Design review of the part built by this model. Coordinates are the model's own, in mm. Give positions to 0.01 mm unless a question says otherwise; leave off trailing zeros. Write each loop counter-clockwise with the first axis right and the second up, starting at its lowest first coordinate (ties: lowest second). Pieces come first, ordered by that corner, then holes. Notation, with made-up numbers: (27.5, 68) -> (35.5, 68) arc R30 cw to (35.5, 107) -> close; hole circle Ø8 at (82, 71). An arc over 180 degrees is marked (long way). Return JSON: item names as keys, results as strings. Group by question number.
Autodesk Inventor part; units mm, degrees
ref_plane "YZ Plane" through (0, 0, 0) normal (1, 0, 0) x (0, 1, 0)
ref_plane "XZ Plane" through (0, 0, 0) normal (0, 1, 0) x (-1, 0, 0)
ref_plane "XY Plane" through (0, 0, 0) normal (0, 0, 1) x (1, 0, 0)
sketch "Sketch1" plane through (0, 0, 0) normal (1, 0, 0) x (0, 1, 0)
  circle A0 centre (0, 0) radius 71
  dimension "d0" = 142
extrude "Extrusion1" add sketch "Sketch1" along normal blind 150
sketch "Sketch2" plane through (150, 0, 0) normal (1, 0, 0) x (0, 0, -1)
  line L0 (0, 0) -> (0, -44.2)
  circle A0 centre (0, 0) radius 71
  line L1 (-55.564, -44.2) -> (55.564, -44.2)
  dimension "d3" = 44.2
extrude "Extrusion2" cut sketch "Sketch2" against normal blind 150 contours A0 L1 picked at (-0.2063, 32.437)
sketch "Sketch3" plane through (150, 0, 0) normal (1, 0, 0) x (0, 0, -1)
  line L0 (0, 0) -> (0, -64.2)
  arc A0 (-55.564, -44.2) -> (55.564, -44.2) centre (0, 0) ccw
  line L1 (-30.3209, -64.2) -> (30.3209, -64.2)
  dimension "d6" = 64.2
sketch "Sketch5" plane through (150, -44.2, 55.564) normal (0, 1, 0) x (1, 0, 0)
  line L0 (-150, 55.564) -> (-75, 55.564)
  line L1 (-75, 55.564) -> (-75, 68.264)
  line L2 (-75, 55.564) -> (-75, 42.864)
  circle A0 centre (-75, 68.264) radius 3
  circle A1 centre (-75, 42.864) radius 3
  line L3 (-75, 68.264) -> (-49.6, 68.264)
  line L4 (-75, 42.864) -> (-49.6, 42.864)
  line L5 (-75, 68.264) -> (-100.4, 68.264)
  line L6 (-75, 42.864) -> (-100.4, 42.864)
  circle A2 centre (-100.4, 68.264) radius 3
  circle A3 centre (-49.6, 68.264) radius 3
  circle A4 centre (-49.6, 42.864) radius 3
  circle A5 centre (-100.4, 42.864) radius 3
  line L7 (-100.4, 42.864) -> (-125.8, 42.864)
  line L8 (-100.4, 68.264) -> (-125.8, 68.264)
  line L9 (-49.6, 68.264) -> (-24.2, 68.264)
  line L10 (-49.6, 42.864) -> (-24.2, 42.864)
  circle A6 centre (-125.8, 68.264) radius 3
  circle A7 centre (-125.8, 42.864) radius 3
  circle A8 centre (-24.2, 68.264) radius 3
  circle A9 centre (-24.2, 42.864) radius 3
  line L11 (-125.8, 68.264) -> (-125.8, 93.664)
  line L12 (-100.4, 68.264) -> (-100.4, 93.664)
  line L13 (-75, 68.264) -> (-75, 93.664)
  line L14 (-75, 68.264) -> (-49.6, 68.264) construction
  line L15 (-49.6, 68.264) -> (-49.6, 93.664)
  line L16 (-24.2, 68.264) -> (-24.2, 93.664)
  line L17 (-125.8, 42.864) -> (-125.8, 17.464)
  line L18 (-100.4, 42.864) -> (-100.4, 17.464)
  line L19 (-75, 42.864) -> (-75, 17.464)
  line L20 (-49.6, 42.864) -> (-49.6, 17.464)
  line L21 (-24.2, 42.864) -> (-24.2, 17.464)
  circle A10 centre (-125.8, 93.664) radius 3
  circle A11 centre (-100.4, 93.664) radius 3
  circle A12 centre (-75, 93.664) radius 3
  circle A13 centre (-49.6, 93.664) radius 3
  circle A14 centre (-24.2, 93.664) radius 3
  circle A15 centre (-24.2, 17.464) radius 3
  circle A16 centre (-49.6, 17.464) radius 3
  circle A17 centre (-75, 17.464) radius 3
  circle A18 centre (-100.4, 17.464) radius 3
  circle A19 centre (-125.8, 17.464) radius 3
  dimension "d9" = 75
  dimension "d10" = 12.7
  dimension "d11" = 12.7
  dimension "d12" = 6
  dimension "d13" = 6
  dimension "d14" = 25.4
  dimension "d15" = 25.4
  dimension "d16" = 25.4
  dimension "d17" = 25.4
  dimension "d18" = 6
  dimension "d19" = 6
  dimension "d20" = 6
  dimension "d21" = 6
  dimension "d22" = 25.4
  dimension "d23" = 25.4
  dimension "d24" = 25.4
  dimension "d25" = 25.4
  dimension "d26" = 6
  dimension "d27" = 6
  dimension "d28" = 6
  dimension "d29" = 6
  dimension "d30" = 25.4
  dimension "d31" = 25.4
  dimension "d32" = 25.4
  dimension "d33" = 90
  dimension "d34" = 25.4
  dimension "d35" = 25.4
  dimension "d36" = 25.4
  dimension "d37" = 25.4
  dimension "d38" = 25.4
  dimension "d39" = 25.4
  dimension "d40" = 25.4
  dimension "d41" = 6
  dimension "d42" = 6
  dimension "d43" = 6
  dimension "d44" = 6
  dimension "d45" = 6
  dimension "d46" = 6
  dimension "d47" = 6
  dimension "d48" = 6
  dimension "d49" = 6
  dimension "d50" = 6
sketch "Sketch6" plane through (150, 0, 0) normal (1, 0, 0) x (0, 0, -1)
  point P0 (0, 0)
extrude "Extrusion4" cut sketch "Sketch3" against normal blind 150
extrude "Extrusion5" cut sketch "Sketch5" against normal blind 10
thread "Thread1"
thread "Thread2"
thread "Thread3"
thread "Thread4"
thread "Thread5"
thread "Thread6"
thread "Thread7"
thread "Thread8"
thread "Thread9"
thread "Thread10"
thread "Thread11"
thread "Thread12"
thread "Thread13"
thread "Thread14"
thread "Thread15"
thread "Thread16"
thread "Thread17"
thread "Thread18"
thread "Thread19"
thread "Thread20"
properties part number "Base"
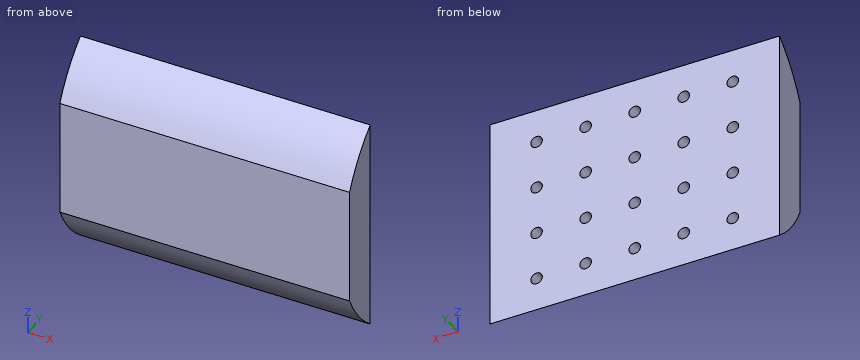
Q1. Take a section at C-C, the plane z = 12.7. Give the boundary of the cut face in (x, y).
Q2. For L1, parallel to X at y = -46.75, z = -38.1; L2, parallel to Z at x = 125.8, y = -48.5; L3, parallel to Z at x = 100.4, y = -46.5, list the stretches that pass through material, from the lowest coordinate up. Write a range as from..to.
Q3. Take a section at B-B, the plane x = 125.8. Give the boundary of the cut face in (y, z), plus the area to 3 significant figures.
Q4. Take a section at A-A, the plane y = -46.5. Count the separate pieces of the cut face and the enclosed holes in it, plus the area to 3 significant figures.
Q5. Take a section at D-D, the plane z = -38.1. Give the boundary of the cut face in (x, y), plus the area to 3 significant figures.
Q6. Insertion check: pin 1 (7 mm diameter, centred on x = 100.4, z = 38.1, fed in from -Y); pin 2 (4 mm diameter, centred on x = 121.5, y = -50.5, fed in from -Z); pin 3 (8 mm diameter, centred on x = 49.6, z = 12.7, fed in from +Y); pin 4 (3 mm diameter, centred on x = 23, z = 12, fed in from +Y). Each pin has a flat end and moves straight along its axis. Give the tip position at first contact, or say it passes through.
Final values:
{
 "1": {"outline": "(0, -64.2) -> (150, -64.2) -> (150, -44.2) -> (128.8, -44.2) -> (128.8, -54.2) -> (122.8, -54.2) -> (122.8, -44.2) -> (103.4, -44.2) -> (103.4, -54.2) -> (97.4, -54.2) -> (97.4, -44.2) -> (78, -44.2) -> (78, -54.2) -> (72, -54.2) -> (72, -44.2) -> (52.6, -44.2) -> (52.6, -54.2) -> (46.6, -54.2) -> (46.6, -44.2) -> (27.2, -44.2) -> (27.2, -54.2) -> (21.2, -54.2) -> (21.2, -44.2) -> (0, -44.2) -> close"},
 "2": {"L1": "x = 0..21.2, 27.2..46.6, 52.6..72, 78..97.4, 103.4..122.8, 128.8..150", "L2": "z = -51.85..-41.1, -35.1..-15.7, -9.7..9.7, 15.7..35.1, 41.1..51.85", "L3": "z = -53.65..-41.1, -35.1..-15.7, -9.7..9.7, 15.7..35.1, 41.1..53.65"},
 "3": {"outline": "(-64.2, -30.32) arc R71 ccw to (-44.2, -55.56) -> (-44.2, -41.1) -> (-54.2, -41.1) -> (-54.2, -35.1) -> (-44.2, -35.1) -> (-44.2, -15.7) -> (-54.2, -15.7) -> (-54.2, -9.7) -> (-44.2, -9.7) -> (-44.2, 9.7) -> (-54.2, 9.7) -> (-54.2, 15.7) -> (-44.2, 15.7) -> (-44.2, 35.1) -> (-54.2, 35.1) -> (-54.2, 41.1) -> (-44.2, 41.1) -> (-44.2, 55.56) arc R71 ccw to (-64.2, 30.32) -> close", "area": "1,560 mm²"},
 "4": {"separate pieces": "1", "enclosed holes": "20", "area": "15,500 mm²"},
 "5": {"outline": "(0, -59.91) -> (150, -59.91) -> (150, -44.2) -> (128.8, -44.2) -> (128.8, -54.2) -> (122.8, -54.2) -> (122.8, -44.2) -> (103.4, -44.2) -> (103.4, -54.2) -> (97.4, -54.2) -> (97.4, -44.2) -> (78, -44.2) -> (78, -54.2) -> (72, -54.2) -> (72, -44.2) -> (52.6, -44.2) -> (52.6, -54.2) -> (46.6, -54.2) -> (46.6, -44.2) -> (27.2, -44.2) -> (27.2, -54.2) -> (21.2, -54.2) -> (21.2, -44.2) -> (0, -44.2) -> close", "area": "2,060 mm²"},
 "6": {"pin 1": "stops at y = -62", "pin 2": "stops at z = -51.85", "pin 3": "stops at y = -44.2", "pin 4": "stops at y = -54.2"}
}
